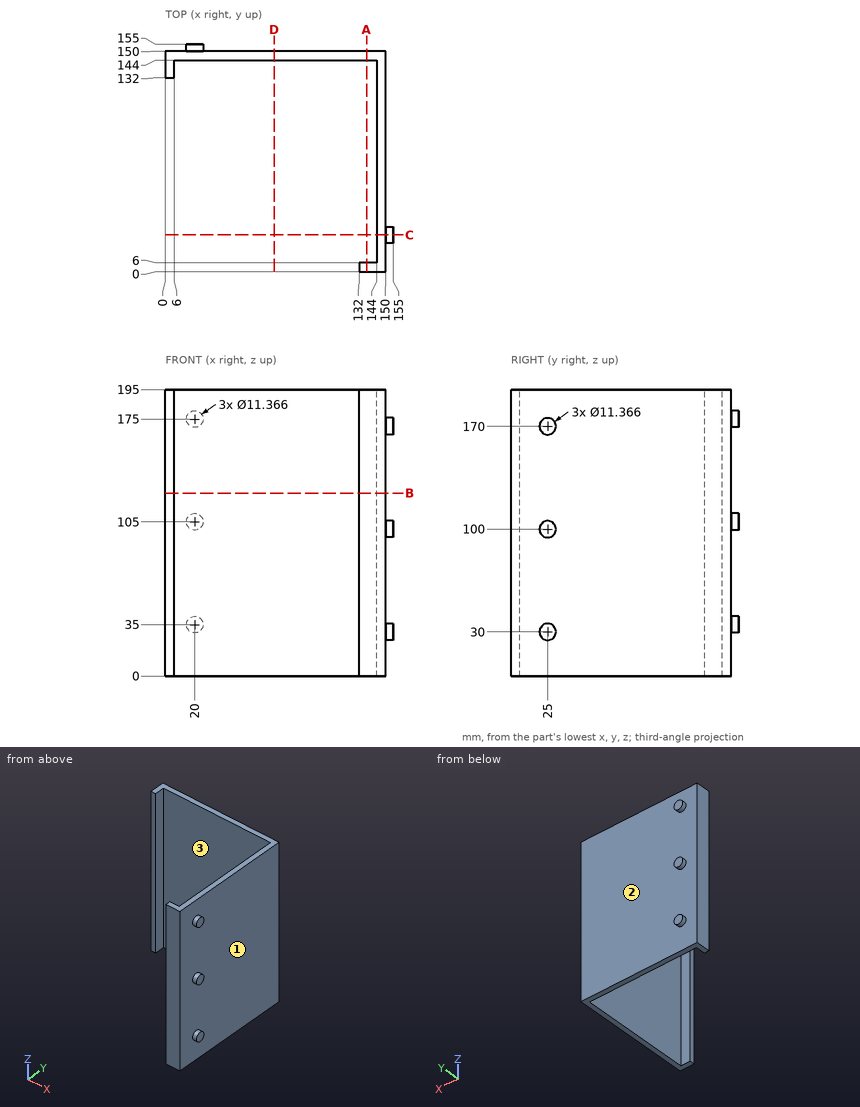
Input: dimensioned drawing with shaded views. Units: mm. Origin: part minimum x, y, z. Round coordinates to 2 decimals unless told otherwise and drop trailing zeros. Order: outer loops, then holes, each group sorted by start corner. A loop starts at its lowest first (then second) coordinate and runs counter-clockwise, first axis right, second up. Notation, with made-up numbers: (88.25, -8) - (110.25, -8) arc R13 ccw to (110.25, 16) - close; hole circle Ø1 at (-37.5, 73). An arc over 180 degrees is marked (long way). Write item = value, one per line. Start each with the question number.
Q1. Pull-direction query (X, two-part tool) for the marked faces 1, 2 and 3; classes: +X half, -X half, draft (parallel to the pull), parting line (faces both ways), or undercut.
Q2. Cut plane A-A on x = 137. Return the cut outline in (y, z), and give its area (3 significant figures).
Q3. Pin query (flat end, axial travel): pin 1 (13 mm diameter, centred on x = 136, z = 71.5, fed in from +Y); pin 2 (6 mm diameter, centred on y = 68, z = 107, fed in from +X); pin 3 (2 mm diameter, centred on y = 70, z = 96, fed in from -X); pin 4 (10 mm diameter, centred on x = 137, y = 51.5, fed in from -Z). Return the tip coordinate at first contact, or that it passes through.
Q4. Cut plane C-C on y = 25. Return the cut outline in (x, z), and give its area (3 significant figures).
Q5. Cut plane B-B on z = 124.5. Return the cut outline in (x, y), and give its area (3 significant figures).
Q6. Ray query, line 1 (Y direction, x = 126.5, z = 73.5); line 2 (X direction, y = 148, z = 128). Return the intervals inside material, ascending. Write a range as from..to.
Q7. Cut plane D-D on x = 74. Return the cut outline in (y, z), and give its area (3 significant figures).
Outcome:
q1.face_1 = +X half
q1.face_2 = draft
q1.face_3 = undercut
q2.outline = (0, 0) - (6, 0) - (6, 195) - (0, 195) - close; (144, 0) - (150, 0) - (150, 195) - (144, 195) - close
q2.area = 2,340 mm^2
q3.pin_1 = 150
q3.pin_2 = 150
q3.pin_3 = 144
q3.pin_4 = through
q4.outline = (144, 0) - (150, 0) - (150, 24.32) - (155, 24.32) - (155, 35.68) - (150, 35.68) - (150, 94.32) - (155, 94.32) - (155, 105.68) - (150, 105.68) - (150, 164.32) - (155, 164.32) - (155, 175.68) - (150, 175.68) - (150, 195) - (144, 195) - close
q4.area = 1,340 mm^2
q5.outline = (0, 132) - (6, 132) - (6, 144) - (144, 144) - (144, 6) - (132, 6) - (132, 0) - (150, 0) - (150, 150) - (0, 150) - close
q5.area = 1,910 mm^2
q6.line_1 = 144..150
q6.line_2 = 0..150
q7.outline = (144, 0) - (150, 0) - (150, 195) - (144, 195) - close
q7.area = 1,170 mm^2
